Autodesk Inventor part; units mm, degrees
ref_plane "YZ Plane" through (0, 0, 0) normal (1, 0, 0) x (0, 1, 0)
ref_plane "XZ Plane" through (0, 0, 0) normal (0, 1, 0) x (-1, 0, 0)
ref_plane "XY Plane" through (0, 0, 0) normal (0, 0, 1) x (1, 0, 0)
sketch "Sketch2" plane through (0, 0, 0) normal (0, 0, 1) x (1, 0, 0)
  line L0 (15, -5) -> (-15, -5)
  line L1 (-15, -5) -> (-15, 5)
  line L2 (-15, 5) -> (15, 5)
  line L3 (15, 5) -> (15, -5)
  line L4 (15, -5) -> (-15, 5) construction
  line L5 (-15, -5) -> (15, 5) construction
  point P0 (0, 0)
  dimension "d192" = 30
  dimension "d193" = 10
extrude "Extrusion1" add sketch "Sketch2" along normal blind 1
sketch "Sketch3" plane through (0, 0, 1) normal (0, 0, 1) x (1, 0, 0)
  circle A0 centre (-10, 0) radius 2.5
  line L0 (15, 5) -> (-15, 5) construction
  line L1 (-15, 5) -> (-15, -5) construction
  line L2 (-15, -5) -> (15, -5) construction
  line L3 (15, -5) -> (15, 5) construction
  point P0 (0, 0)
  dimension "d196" = 5
  dimension "d197" = 10
extrude "Extrusion2" cut sketch "Sketch3" against normal blind 1
sketch "Sketch4" plane through (0, 0, 1) normal (0, 0, 1) x (1, 0, 0)
  circle A0 centre (10, 0) radius 2.5
  point P0 (0, 0)
  dimension "d200" = 5
  dimension "d201" = 10
extrude "Extrusion3" cut sketch "Sketch4" against normal blind 1
sketch "Sketch5" plane through (0, 0, 1) normal (0, 0, 1) x (1, 0, 0)
  line L0 (-15, -5) -> (15, -5) construction
  line L1 (-15, -5) -> (15, -5)
  line L2 (-12, -5) -> (-10.5441, -9)
  line L3 (-10.5441, -9) -> (-9.0882, -5)
  point P0 (0, 0)
  dimension "d204" = 4
  dimension "d205" = 70
  dimension "d206" = 70
  dimension "d207" = 12
extrude "Extrusion4" add sketch "Sketch5" against normal blind 1
pattern_linear "Rectangular Pattern1" count 6 spacing 4 along (1, 0, 0) of "Extrusion4"
fillet "Fillet1" radius 2 1 edges at (-15, 5, 0.5)
fillet "Fillet2" radius 2 1 edges at (15, 5, 0.5)
fillet "Fillet3" radius 2 1 edges at (15, -5, 0.5)
fillet "Fillet4" radius 1 1 edges at (-15, -5, 0.5)
properties part number "50_sierra-01"
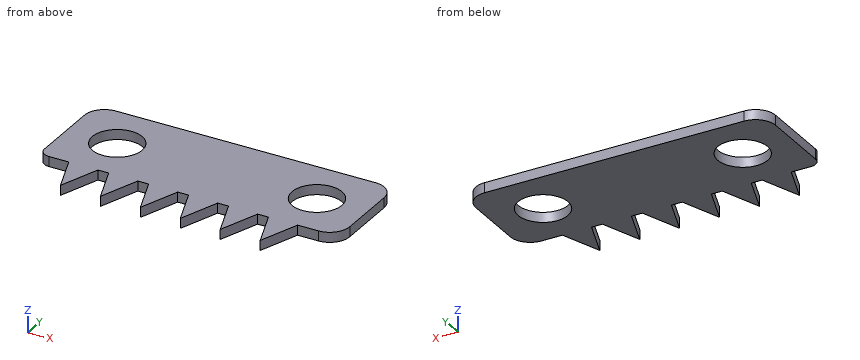
The listing builds one solid part. Answer for the finished solid, in the listing's coordinates (mm). Coordinates: 2 decimals unless noted, no trailing zeros. Write each loop counter-clockwise with the first axis right and the second up, starting at its lowest first coordinate (ties: lowest second). Pieces come first, ordered by that corner, then holes. Notation, with made-up numbers: (55, 17.25) - (67, 17.25) arc R23 cw to (67, 28.25) - close; hole circle Ø8 at (77, -27.75). An arc over 180 degrees is marked (long way). Return JSON: item names as keys, results as strings. Group by question number.
Q1. A flat-ended cylindrical pin translates along its axis: pin 1 Ø0.5 at (x, z) = (-4.5, 0.5) entering from -Y. Find the tip coordinate at first contact, or state that the pin passes through.
Q2. The part is cut by section D-D on y = -5.75. Write down the section's boundary in (x, z), and give its area (3 significant figures).
Q3. The part is cut by section B-B on z = 0.35. Write down the section's boundary in (x, y), and give its area (3 significant figures).
Q4. The part is cut by section C-C on x = -10. Write down the section's boundary in (y, z).
Q5. The part is cut by section A-A on y = 0. Write down the section's boundary in (x, z).
Q6. Find the intervals of material crossed by line 1 along X through (y, z) = (-2, 0.85); line 2 along Y through (x, z) = (-0.75, 0.75); line 3 along X through (y, z) = (-7.25, 0.2), in increasing order. Write a range as [from, to].
Evaluation:
{
 "1": {"pin 1": "stops at y = -5"},
 "2": {"outline": "(-11.73, 0) - (-9.36, 0) - (-9.36, 1) - (-11.73, 1) - close; (-7.73, 0) - (-5.36, 0) - (-5.36, 1) - (-7.73, 1) - close; (-3.73, 0) - (-1.36, 0) - (-1.36, 1) - (-3.73, 1) - close; (0.27, 0) - (2.64, 0) - (2.64, 1) - (0.27, 1) - close; (4.27, 0) - (6.64, 0) - (6.64, 1) - (4.27, 1) - close; (8.27, 0) - (10.64, 0) - (10.64, 1) - (8.27, 1) - close", "area": "14.2 mm2"},
 "3": {"outline": "(-15, -4) arc R1 ccw to (-14, -5) - (-12, -5) - (-10.54, -9) - (-9.09, -5) - (-8, -5) - (-6.54, -9) - (-5.09, -5) - (-4, -5) - (-2.54, -9) - (-1.09, -5) - (0, -5) - (1.46, -9) - (2.91, -5) - (4, -5) - (5.46, -9) - (6.91, -5) - (8, -5) - (9.46, -9) - (10.91, -5) - (13, -5) arc R2 ccw to (15, -3) - (15, 3) arc R2 ccw to (13, 5) - (-13, 5) arc R2 ccw to (-15, 3) - close; hole circle Ø5 at (-10, 0); hole circle Ø5 at (10, 0)", "area": "293 mm2"},
 "4": {"outline": "(-7.51, 0) - (-2.5, 0) - (-2.5, 1) - (-7.51, 1) - close; (2.5, 0) - (5, 0) - (5, 1) - (2.5, 1) - close"},
 "5": {"outline": "(-15, 0) - (-12.5, 0) - (-12.5, 1) - (-15, 1) - close; (-7.5, 0) - (7.5, 0) - (7.5, 1) - (-7.5, 1) - close; (12.5, 0) - (15, 0) - (15, 1) - (12.5, 1) - close"},
 "6": {"line 1": "x = [-15, -11.5], [-8.5, 8.5], [11.5, 15]", "line 2": "y = [-5, 5]", "line 3": "x = [-11.18, -9.91], [-7.18, -5.91], [-3.18, -1.91], [0.82, 2.09], [4.82, 6.09], [8.82, 10.09]"}
}
